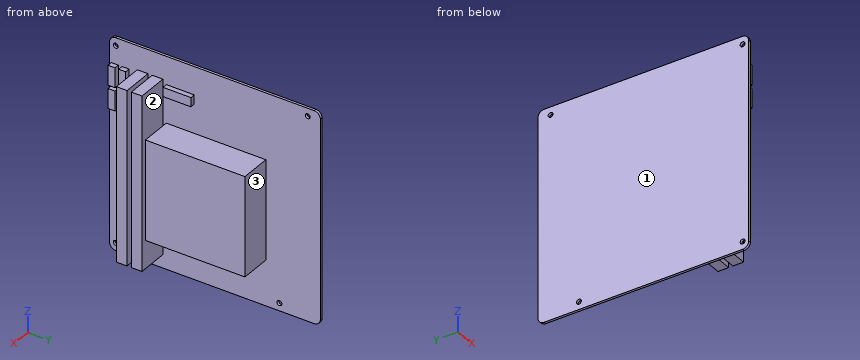
```python
from build123d import *

# Parameters (mm, degrees)
F0_R     = 1.98
F1_DEPTH = 2
F3_ANGLE = -90
F4_W     = 5.638488
F4_H     = 15.871309
F4_W_2   = 5.638487
F5_DEPTH = 4
F4_W_3   = 4.60542
F4_H_2   = 27.714742
F6_DEPTH = 4
F4_W_4   = 22.524819
F4_H_3   = 7.381014
F7_DEPTH = 4
F4_W_5   = 80.340352
F4_H_4   = 80.123208
F8_DEPTH = 25
F4_W_6   = 8.616418
F4_H_5   = 140.016765
F4_W_7   = 8.616417
F9_DEPTH = 25


with BuildPart() as f1:
    # F0 (on Right) → F1 (new body)
    with BuildSketch(Plane.YZ):
        with BuildLine():
            Line((-80, -85), (80, -85))
            ThreePointArc((80, -85), (83.535534, -83.535534), (85, -80))
            Line((85, -80), (85, 80))
            ThreePointArc((85, 80), (83.535534, 83.535534), (80, 85))
            Line((80, 85), (-80, 85))
            ThreePointArc((-80, 85), (-83.535534, 83.535534), (-85, 80))
            Line((-85, 80), (-85, -80))
            ThreePointArc((-85, -80), (-83.535534, -83.535534), (-80, -85))
        make_face()
        with Locations((-78.65, -80.1)):
            Circle(F0_R, mode=Mode.SUBTRACT)
        with Locations((78.83, -80.1)):
            Circle(F0_R, mode=Mode.SUBTRACT)
        with Locations((-78.65, 74.84)):
            Circle(F0_R, mode=Mode.SUBTRACT)
        with Locations((78.83, 51.98)):
            Circle(F0_R, mode=Mode.SUBTRACT)
    extrude(amount=F1_DEPTH)


with BuildPart() as f1_1:
    # F3: moved
    add(f1.part.rotate(Axis((1.078181, 0, 0), (1, 0, 0)), F3_ANGLE))

    # F4 (on face) → F5 (join)
    with BuildSketch(Plane.YZ.offset(2)):
        with Locations((-72.176602, 55.920038)):
            Rectangle(F4_W, F4_H)
        with Locations((-80.823529, 55.920038)):
            Rectangle(F4_W_2, F4_H)
        with Locations((-80.823529, 37.344094)):
            Rectangle(F4_W_2, F4_H)
        with Locations((-72.176602, 37.344094)):
            Rectangle(F4_W, F4_H)
    extrude(amount=F5_DEPTH)

    # F4 (on face) → F6 (join)
    with BuildSketch(Plane.YZ.offset(2)):
        with Locations((-72.246823, 14.365959)):
            Rectangle(F4_W_3, F4_H_2)
    extrude(amount=F6_DEPTH)

    # F4 (on face) → F7 (join)
    with BuildSketch(Plane.YZ.offset(2)):
        with Locations((-28.006542, 58.70362)):
            Rectangle(F4_W_4, F4_H_3)
    extrude(amount=F7_DEPTH)

    # F4 (on face) → F8 (join)
    with BuildSketch(Plane.YZ.offset(2)):
        with Locations((0.842279, -8.411627)):
            Rectangle(F4_W_5, F4_H_4)
    extrude(amount=F8_DEPTH)

    # F4 (on face) → F9 (join)
    with BuildSketch(Plane.YZ.offset(2)):
        with Locations((-58.420569, -4.278883)):
            Rectangle(F4_W_6, F4_H_5)
        with Locations((-46.367261, -4.278883)):
            Rectangle(F4_W_7, F4_H_5)
    extrude(amount=F9_DEPTH)


solid = f1_1.part
```
For this review, take the finished solid that the model builds, in its own axes (mm). Face numbers are marked on the shaded views. A direction names the side the tool comes from. Give positions to 0.01 mm unless a question says otherwise; leave off trailing zeros. Write each loop counter-clockwise with the first axis right and the second up, starting at its lowest first coordinate (ties: lowest second). Pieces come first, ordered by that corner, then holes.
Item 1: Take a section at B-B (x = 21.75). Give the boundary of the cut face in (y, z).
Item 2: Wall thickness on probe 1 along Y at (x, z) = (13.25, -32); probe 2 along Y at (x, z) = (21, -51.5); probe 3 along X at (y, z) = (-11.5, 54.5): over which ranges is each line inside the solid? List them lowest first.
Item 3: Take a section at D-D (z = 39.5). Give the boundary of the cut face in (x, y).
Item 4: Machinability: for the marked faces 1, 2 and 3, which of the approach directions +Z, -Z, +X, -X, +Y, -Y give a long, thin tool a straight path to every point of the face, cutting with its end or side? Answer none if there is none.
Item 5: Take a section at A-A (y = 51.98). Give the boundary of the cut face in (x, z), and give its area (3 significant figures).
Item 6: Insertion check: P1, Ø1.2, axis at x = 3.5, y = -73, coming from the -Z side; P2, Ø2.5, axis at x = 13.5, y = -47, coming from the +Z side; P3, Ø7, axis at x = 10.5, y = -58, coming from the -Z side; P4, Ø2.5, axis at y = 51.98, z = -78.83, coming from the +X side. Each pin has a flat end and moves straight along its axis. Give the tip position at first contact, or say it passes through.
Item 7: Take a section at C-C (y = 33.5). Give the boundary of the cut face in (x, z), and give its area (3 significant figures).
Established:
1. outline: (-62.73, -74.29) - (-54.11, -74.29) - (-54.11, 65.73) - (-62.73, 65.73) - close; (-50.68, -74.29) - (-42.06, -74.29) - (-42.06, 65.73) - (-50.68, 65.73) - close; (-39.33, -48.47) - (41.01, -48.47) - (41.01, 31.65) - (-39.33, 31.65) - close
2. probe 1: y = -62.73 to -54.11, -50.68 to -42.06, -39.33 to 41.01
2. probe 2: y = -62.73 to -54.11, -50.68 to -42.06
2. probe 3: x = 0 to 2
3. outline: (0, -85) - (2, -85) - (2, -83.64) - (6, -83.64) - (6, -78) - (2, -78) - (2, -75) - (6, -75) - (6, -69.36) - (2, -69.36) - (2, -62.73) - (27, -62.73) - (27, -54.11) - (2, -54.11) - (2, -50.68) - (27, -50.68) - (27, -42.06) - (2, -42.06) - (2, 85) - (0, 85) - close
4. face 1: +Z, -Z, -X, +Y, -Y
4. face 2: +Z, -Z, +X
4. face 3: +Z, -Z, +X, +Y
5. outline: (0, -85) - (2, -85) - (2, -80.81) - (0, -80.81) - close; (0, -76.85) - (2, -76.85) - (2, 85) - (0, 85) - close
5. area: 332 mm2
6. P1: stops at z = 0.51
6. P2: stops at z = 65.73
6. P3: stops at z = -74.29
6. P4: passes through
7. outline: (0, -85) - (2, -85) - (2, -48.47) - (27, -48.47) - (27, 31.65) - (2, 31.65) - (2, 85) - (0, 85) - close
7. area: 2,340 mm2
